Could you check a few things on this model? Use its own coordinates, in mm. Round coordinates to 2 decimals unless told otherwise and drop trailing zeros. Loops run counter-clockwise (first coordinate to the right, second up) from the corner with the lowest first, then second, coordinate; pieces in that order, holes last. Notation, with made-up numbers: (42.5, 89) - (92.5, 89) arc R11 ccw to (92.5, 105) - close; hole circle Ø8 at (43, -35). An arc over 180 degrees is marked (long way). Answer as CSV lines item,"result". Start each with the question number.
1) Please list where these lines run through material, in increasing order: line 1 along X through (y, z) = (0, 1.75); line 2 along Y through (x, z) = (0, 0.9); line 3 along X through (y, z) = (-237, 0.7).
2) I'm going to push flat-ended pins straight in: pin 1 Ø1.5 at (y, z) = (-284.5, 1) entering from +X; pin 2 Ø1.5 at (x, z) = (-227.5, 1.5) entering from -Y; pin 3 Ø4 at (x, y) = (155.5, 574.5) entering from -Z. Where does each tip first touch, or does it pass through?
3) Suppose I cut it at D-D, the plane x = -598. Write out the boundary of the cut face in (y, z) (3 decimals).
4) Suppose I cut it at B-B, the plane x = 0. Write out the boundary of the cut face in (y, z) (3 decimals), then the cut area to 3 significant figures.
5) We'd pull the mould along X, two halves only. Please class faces 1 (the face through (321.404, -409.07, 1.565)), 2 (the face through (49.592, -11.012, 1.61)), 3 (the face through (-60, 114, 0)): pulls with the +X half, pulls with the -X half, needs draft (parallel to the pull), parting line crosses it, or undercut.
6) Suppose I cut it at C-C, the plane y = -326. Write out the boundary of the cut face in (x, z) (3 decimals), then the cut area to 3 significant figures.
Autodesk Inventor part; units mm, degrees
ref_plane "YZ Plane" through (0, 0, 0) normal (1, 0, 0) x (0, 1, 0)
ref_plane "XZ Plane" through (0, 0, 0) normal (0, 1, 0) x (-1, 0, 0)
ref_plane "XY Plane" through (0, 0, 0) normal (0, 0, 1) x (1, 0, 0)
sketch "Sketch1" plane through (0, 0, 0) normal (0, 0, 1) x (1, 0, 0)
  circle A0 centre (0, 0) radius 69.85 construction
  line L0 (69.85, 0) -> (34.925, -60.4919) construction
  line L1 (34.925, -60.4919) -> (-34.925, -60.4919) construction
  line L2 (-34.925, -60.4919) -> (-69.85, 0) construction
  line L3 (-69.85, 0) -> (-34.925, 60.4919) construction
  line L4 (-34.925, 60.4919) -> (34.925, 60.4919) construction
  line L5 (34.925, 60.4919) -> (69.85, 0) construction
  line L6 (69.85, 0) -> (69.85, 777.875) construction
  line L7 (0, 60.4919) -> (0, -60.4919) construction
  line L8 (-69.85, 0) -> (69.85, 0) construction
  arc A1 (69.85, 777.875) -> (-319.0875, 673.6595) centre (69.85, 0) ccw
  arc A2 (-319.0875, 673.6595) -> (-673.1, 60.4919) centre (34.925, 60.4919) ccw
  arc A3 (-673.1, 60.4919) -> (-354.0125, -492.1839) centre (-34.925, 60.4919) ccw
  arc A4 (-354.0125, -492.1839) -> (214.3125, -492.1839) centre (-69.85, 0) ccw
  arc A5 (214.3125, -492.1839) -> (463.55, -60.4919) centre (-34.925, -60.4919) ccw
  arc A6 (463.55, -60.4919) -> (458.7952, 3.175) centre (34.925, -60.4919) ccw
  line L9 (458.7952, 3.175) -> (571.5, 3.175)
  line L10 (571.5, 3.175) -> (571.5, 777.875)
  line L11 (69.85, 777.875) -> (571.5, 777.875)
  line L12 (571.5, 3.175) -> (400.325, -303.4625)
  dimension "d0" = 777.875
  dimension "d1" = 139.7
  dimension "d2" = 571.5
  dimension "d3" = 774.7
  dimension "d5" = 498.475
extrude "Extrusion1" add sketch "Sketch1" along normal blind 3.175
hole "Hole1" at (0, 0, 0) direction (0, 0, 1) diameter 101.6 end through all
ref_plane "Work Plane1" through (0, 0, 1833.3831) normal (-1, 0, 0) x (0, 0, 1)
ref_plane "Work Plane2" through (0, 0, 1833.3831) normal (0, -1, 0) x (0, 0, 1)
ref_plane "Work Plane3" through (0, 0, 1833.3831) normal (0.7071, -0.7071, 0) x (0, 0, 1)
ref_plane "Work Plane4" through (0, 0, 1833.3831) normal (-0.7071, -0.7071, 0) x (0, 0, 1)
properties part number "drive side sheet" material "Steel, Mild"
Filled sheet:
1,line 1,"-670.23 to -50.8, 50.8 to 569.73"
1,line 2,"-564.02 to -50.8, 50.8 to 774.73"
1,line 3,"-599.52 to 437.43"
2,pin 1,"x = 411.33"
2,pin 2,"y = -546.24"
2,pin 3,"z = 0"
3,outline,"(-239.864, 0) - (377.833, 0) - (377.833, 3.175) - (-239.864, 3.175) - close"
4,outline,"(-564.016, 0) - (-50.8, 0) - (-50.8, 3.175) - (-564.016, 3.175) - close; (50.8, 0) - (774.733, 0) - (774.733, 3.175) - (50.8, 3.175) - close"
4,area,"3,930 mm²"
5,face 1,"pulls with the +X half"
5,face 2,"undercut"
5,face 3,"needs draft"
6,outline,"(-542.755, 0) - (386.955, 0) - (386.955, 3.175) - (-542.755, 3.175) - close"
6,area,"2,950 mm²"
